Autodesk Inventor part; units mm, degrees
ref_plane "YZ Plane" through (0, 0, 0) normal (1, 0, 0) x (0, 1, 0)
ref_plane "XZ Plane" through (0, 0, 0) normal (0, 1, 0) x (-1, 0, 0)
ref_plane "XY Plane" through (0, 0, 0) normal (0, 0, 1) x (1, 0, 0)
sketch "Sketch1" plane through (0, 0, 0) normal (0, 0, 1) x (1, 0, 0)
  circle A0 centre (0, 0) radius 5
  dimension "d0" = 10
extrude "Extrusion1" add sketch "Sketch1" along normal blind 18.75
sketch "Sketch2" plane through (0, 0, 18.75) normal (0, 0, 1) x (1, 0, 0)
  circle A0 centre (0, 0) radius 5
  circle A1 centre (0, 0) radius 4.625
  dimension "d3" = 9.25
extrude "Extrusion2" cut sketch "Sketch2" against normal blind 8
sketch "Sketch3" plane through (0, 0, 18.75) normal (0, 0, 1) x (1, 0, 0)
  circle A0 centre (0, 0) radius 1.5
  dimension "d6" = 3
extrude "Extrusion3" cut sketch "Sketch3" against normal blind 50
sketch "Sketch4" plane through (0, 0, 0) normal (0, 0, -1) x (-1, 0, 0)
  circle A0 centre (0, 0) radius 3.375
  circle A1 centre (0, 0) radius 5
  dimension "d9" = 6.75
  dimension "d10" = 10
extrude "Extrusion4" cut sketch "Sketch4" against normal blind 8.25
sketch "Sketch5" plane through (0, 0, 8.25) normal (0, 0, -1) x (-1, 0, 0)
  circle A0 centre (0, 0) radius 3.375
  circle A1 centre (0, 0) radius 3.375
  circle A2 centre (0, 0) radius 5
  dimension "d13" = 6.75
  dimension "d14" = 10
thread "Thread1"
thread "Thread2"
sketch "Sketch6" plane through (0, 0, 8.25) normal (0, 0, -1) x (-1, 0, 0)
  circle A0 centre (0, 0) radius 3.375
  circle A1 centre (0, 0) radius 5
extrude "Extrusion5" cut sketch "Sketch6" against normal blind 1.25
properties part number "cuvette_holder_fiber_optics_connector"
Work out the finished part from the listing and answer in its coordinate system (mm). A direction names the side the tool comes from. Round coordinates to 2 decimals unless told otherwise and drop trailing zeros. Order: outer loops, then holes, each group sorted by start corner. A loop starts at its lowest first (then second) coordinate and runs counter-clockwise, first axis right, second up. Notation, with made-up numbers: M 88.25,28 L 128.25,28 A18 cw 128.25,49 Z; hole C -39.75,68 d10. An arc over 180 degrees is marked long. Put each result on its own line as item: value. Start each with the question number.
Q1. A tool of negligible diameter and unlimited length cuts with its end or side. For faces 1 (the cylindrical face through (0.7, -3.3, 4.7)), 2 (the flat face through (1.5, -0.7, 0)), from which of +Z, -Z, +X, -X, +Y, -Y can it reach the whole face along a straight path? Write none if from no direction.
Q2. Section D-D, the plane y = 2.25 is taken. Write down the section's boundary in (x, z), and give its area (3 significant figures).
Q3. Straight lines are drawn through the part: L1, parallel to Y at x = 0, z = 11.5 (3 decimals); L2, parallel to Y at x = 0, z = 7 (3 decimals); L3, parallel to X at y = -0.5, z = 4.25. For each, find the intervals that lie inside material, in ascending order. Write a range as [from, to].
Q4. Section A-A, the plane x = 0 is taken. Write down the section's boundary in (y, z) (3 decimals), and give its area (3 significant figures).
Q5. For a pull along X with two mould halves and no side action, classify faces 3 (the flat face through (2, 0, 18.75)), 4 (the cylindrical face through (-1.5, 0.07, 9.51)), 5 (the cylindrical face through (-1.003, -4.515, 14.806)) as pulls with the +X half, pulls with the -X half, needs draft (parallel to the pull), parting line crosses it, or undercut.
Q6. Flat-ended cylindrical pins translate along their axes: pin 1 (5 mm diameter, centred on y = 3.5, z = 6, fed in from +X); pin 2 (2 mm diameter, centred on y = 2, z = 10, fed in from -X); pin 3 (5 mm diameter, centred on y = -1, z = 2.5, fed in from -X) (3 decimals). Find the tip coordinate at first contact, or state that the pin passes through.
Q7. Section B-B, the plane y = -1.25 is taken. Write down the section's boundary in (x, z).
Q8. Section C-C, the plane z = 16 is taken. Write down the section's boundary in (x, y) (3 decimals), and give its area (3 significant figures).
Findings below:
1. face 1: -Z
1. face 2: -Z, +X, -X, +Y, -Y
2. outline: M -4.47,9.5 L -2.52,9.5 L -2.52,0 L 2.52,0 L 2.52,9.5 L 4.47,9.5 L 4.47,10.75 L 4.04,10.75 L 4.04,18.75 L -4.04,18.75 L -4.04,10.75 L -4.47,10.75 Z
2. area: 124 mm^2
3. L1: y = [-4.625, -1.5], [1.5, 4.625]
3. L2: y = [-3.375, -1.5], [1.5, 3.375]
3. L3: x = [-3.34, -1.41], [1.41, 3.34]
4. outline: M -5,9.5 L -3.375,9.5 L -3.375,0 L -1.5,0 L -1.5,18.75 L -4.625,18.75 L -4.625,10.75 L -5,10.75 Z; M 1.5,0 L 3.375,0 L 3.375,9.5 L 5,9.5 L 5,10.75 L 4.625,10.75 L 4.625,18.75 L 1.5,18.75 Z
4. area: 94.4 mm^2
5. face 3: needs draft
5. face 4: undercut
5. face 5: parting line crosses it
6. pin 1: stops at x = 3.22
6. pin 2: stops at x = -4.9
6. pin 3: stops at x = -3.375
7. outline: M -4.84,9.5 L -3.13,9.5 L -3.13,0 L -0.83,0 L -0.83,18.75 L -4.45,18.75 L -4.45,10.75 L -4.84,10.75 Z; M 0.83,0 L 3.13,0 L 3.13,9.5 L 4.84,9.5 L 4.84,10.75 L 4.45,10.75 L 4.45,18.75 L 0.83,18.75 Z
8. outline: C 0,0 d9.25; hole C 0,0 d3
8. area: 60.1 mm^2
